Source: CAD feature listing. Evaluate the final solid. Frame: model axes, mm. Round coordinates to 2 decimals unless told otherwise and drop trailing zeros. Loops run counter-clockwise (first coordinate to the right, second up) from the corner with the lowest first, then second, coordinate; pieces in that order, holes last. Notation, with made-up numbers: M -26.5,5 L 3.5,5 A27 ccw 3.5,27 Z; hole C 40.5,-32.5 d8. An arc over 180 degrees is marked long. Answer as a JSON object with one key per item and string values.
from build123d import *

# Parameters (mm, degrees)
F2_R          = 17.5
F3_DEPTH      = 40.001
F3_DEPTH_BACK = 40.001
F4_R          = 21.5
F5_DEPTH      = 40.001
F5_DEPTH_BACK = 40.001


with BuildPart() as f1:
    # F0 (on Front) → F1 (revolve)
    with BuildSketch(Plane.XZ):
        with BuildLine():
            Line((0, 37), (0, 40))
            ThreePointArc((0, 40), (-40, 0), (0, -40))
            Line((0, -40), (0, -37))
            ThreePointArc((0, -37), (-37, 0), (0, 37))
        make_face()
    revolve(axis=Axis((0, 0, -38.5), (0, 0, -1)))

    # F2 (on Front) → F3 (cut, two sides)
    with BuildSketch(Plane.XZ) as f3_sk:
        Circle(F2_R)
    extrude(amount=F3_DEPTH, mode=Mode.SUBTRACT)
    extrude(f3_sk.sketch, amount=-F3_DEPTH_BACK, mode=Mode.SUBTRACT)

    # F4 (on Top) → F5 (cut, two sides)
    with BuildSketch(Plane.XY) as f5_sk:
        Circle(F4_R)
    extrude(amount=F5_DEPTH, mode=Mode.SUBTRACT)
    extrude(f5_sk.sketch, amount=-F5_DEPTH_BACK, mode=Mode.SUBTRACT)


solid = f1.part
Item 1: Section B-B on y = 0. Return the cut outline in (x, z).
Answer sheet:
{"outline": "M -21.5,-33.73 L -21.5,-30.11 A37 cw -21.5,30.11 L -21.5,33.73 A40 ccw Z; M 21.5,-33.73 A40 ccw 21.5,33.73 L 21.5,30.11 A37 cw 21.5,-30.11 Z"}
Item 2: Line query: probe 1 along Z at (x, y) = (34, -5.5); probe 2 along X at (y, z) = (33.75, 0); probe 3 along Y at (x, z) = (-25, 3.5). Output: solid intervals per line, ascending. Write a range as from..to.
Answer sheet:
{"probe 1": "z = -20.34..-13.52, 13.52..20.34", "probe 2": "x = -21.47..-17.5, 17.5..21.47", "probe 3": "y = -31.03..-27.05, 27.05..31.03"}
Item 3: Section A-A on x = 0. Return the cut outline in (y, z), then the cut area to 3 significant figures.
Answer sheet:
{"outline": "M -35.97,-17.5 A40 ccw -21.5,-33.73 L -21.5,-30.11 A37 cw -32.6,-17.5 Z; M -35.97,17.5 L -32.6,17.5 A37 cw -21.5,30.11 L -21.5,33.73 A40 ccw Z; M 21.5,-33.73 A40 ccw 35.97,-17.5 L 32.6,-17.5 A37 cw 21.5,-30.11 Z; M 21.5,30.11 A37 cw 32.6,17.5 L 35.97,17.5 A40 ccw 21.5,33.73 Z", "area": "234 mm²"}
Item 4: Section D-D on x = -8.5. Return the cut outline in (y, z).
Answer sheet:
{"outline": "M -35.97,-15.3 A39.09 ccw -19.75,-33.73 L -19.75,-30.11 A36.01 cw -32.6,-15.3 Z; M -35.97,15.3 L -32.6,15.3 A36.01 cw -19.75,30.11 L -19.75,33.73 A39.09 ccw Z; M 19.75,-33.73 A39.09 ccw 35.97,-15.3 L 32.6,-15.3 A36.01 cw 19.75,-30.11 Z; M 19.75,30.11 A36.01 cw 32.6,15.3 L 35.97,15.3 A39.09 ccw 19.75,33.73 Z"}
Item 5: Pull-direction query (Z, two-part tool) for faces 1 (the cylindrical face through (-15.846, 14.531, -31.896)), 2 (the cylindrical face through (-13.887, -34.261, -10.648)); classes: pulls with the +Z half, pulls with the -Z half, needs draft (parallel to the pull), parting line crosses it, or undercut.
Answer sheet:
{"face 1": "needs draft", "face 2": "undercut"}
Item 6: Section C-C on z = -25. Return the cut outline in (x, y), then the cut area to 3 significant figures.
Answer sheet:
{"outline": "C 0,0 d62.45; hole C 0,0 d54.55", "area": "726 mm²"}
Item 7: Contact query for flat-ended pins moving along their axis: pin 1 Ø1 at (y, z) = (8, 22) entering from -X; pin 2 Ø2 at (x, y) = (25.5, 16.5) entering from +Z; pin 3 Ø12 at (y, z) = (-12, 24.5) entering from -X. Output: stop coordinate, or through.
Answer sheet:
{"pin 1": "stops at x = -32.79", "pin 2": "stops at z = 27.15", "pin 3": "stops at x = -33.87"}
